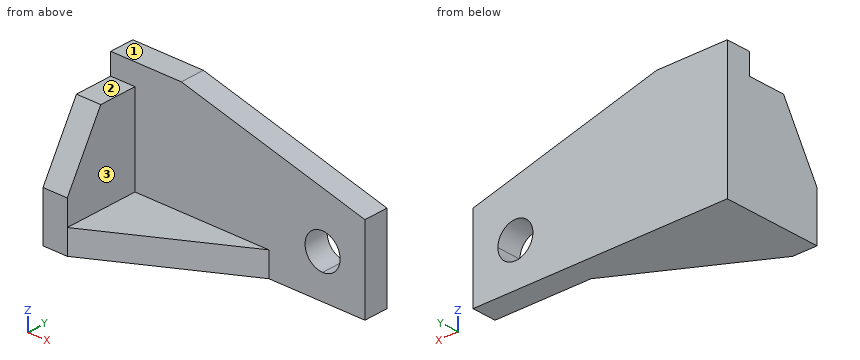
from build123d import *

# Parameters (mm, degrees)
F1_DEPTH  = 10.922
F2_W      = 10.922
F2_H      = 50.8
F3_DEPTH  = 33.528
F4_W      = 60.198
F4_H      = 10.922
F5_DEPTH  = 33.528
F7_DEPTH  = 25.4
F9_DEPTH  = 10.923
F11_DEPTH = 10.923


with BuildPart() as f1:
    # F0 (on Front) → F1 (new body)
    with BuildSketch(Plane.XZ):
        Polygon((-61.109246, 15.510071), (-92.859246, 15.510071), (-92.859246, -44.687929), (21.440754, -44.687929), (21.440754, -6.609135), align=None)
    extrude(amount=F1_DEPTH)

    # F2 (on face) → F3 (join)
    with BuildSketch(Plane.XZ.offset(10.922)):
        with Locations((-87.398246, -19.287929)):
            Rectangle(F2_W, F2_H)
    extrude(amount=F3_DEPTH)

    # F4 (on face) → F5 (join)
    with BuildSketch(Plane.XZ.offset(10.922)):
        with Locations((-51.838246, -39.226929)):
            Rectangle(F4_W, F4_H)
    extrude(amount=F5_DEPTH)

    # F6 (on face) → F7 (cut)
    with BuildSketch(Plane.XY.offset(-33.765929)):
        Polygon((-21.739246, -10.922), (-81.937246, -44.45), (-21.739246, -44.45), align=None)
    extrude(amount=-F7_DEPTH, mode=Mode.SUBTRACT)

    # F8 (on face) → F9 (cut, through all)
    with BuildSketch(Plane.XZ.offset(10.922)):
        with BuildLine():
            ThreePointArc((10.264754, -25.637929), (-3.177005, -20.070171), (2.390754, -33.511929))
            Line((2.390754, -33.511929), (2.390754, -25.637929))
            Line((2.390754, -25.637929), (10.264754, -25.637929))
        make_face()
        with BuildLine():
            Line((2.390754, -25.637929), (2.390754, -33.511929))
            ThreePointArc((2.390754, -33.511929), (7.958513, -31.205688), (10.264754, -25.637929))
            Line((10.264754, -25.637929), (2.390754, -25.637929))
        make_face()
    extrude(amount=-F9_DEPTH, mode=Mode.SUBTRACT)

    # F10 (on face) → F11 (cut, through all)
    with BuildSketch(Plane.YZ.offset(-81.937246)):
        Polygon((-44.45, 6.112071), (-44.45, -22.589929), (-27.878893, 6.112071), align=None)
    extrude(amount=-F11_DEPTH, mode=Mode.SUBTRACT)


solid = f1.part
Read the model definition and answer for the solid it produces. Units are mm, in the model's axes. Face numbers are marked on the shaded views. A direction names the side the tool comes from. Round coordinates to 2 decimals unless told otherwise and drop trailing zeros. Order: outer loops, then holes, each group sorted by start corner. A loop starts at its lowest first (then second) coordinate and runs counter-clockwise, first axis right, second up. Notation, with made-up numbers: (-34, -6) - (3, -6) arc R24 ccw to (3, 6) - close; hole circle Ø5 at (-4.75, 44). An arc over 180 degrees is marked (long way). Use one line per item in the form item = value. Start each with the question number.
(1) The part is cut by section C-C (y = -8). Give the vertices of the cut face in (x, z).
(2) Find the intervals of material crossed by line 1 along Z through (x, y) = (-59.5, -25.5); line 2 along Y through (x, z) = (-15.5, -6); line 3 along X through (y, z) = (-13, -19), in increasing order. Write a range as from..to.
(3) The part is cut by section B-B (z = -32). Give the vertices of the cut face in (x, y).
(4) For the marked faces 1, 2 and 3, determine the directions among +Z, -Z, +X, -X, +Y, -Y from which every point of the face is accessible in a straight line to the end or side of a thin tool.
(5) The part is cut by section A-A (x = 8). Give the vertices of the cut face in (y, z), then the cut area to 3 significant figures.
(6) The part is cut by section D-D (z = -13). Give the vertices of the cut face in (x, y).
(7) Flat-ended cylindrical pins translate along their axes: pin 1 Ø12 at (x, y) = (-51.5, -32) entering from +Z; pin 2 Ø1.5 at (x, z) = (-29.5, -29.5) entering from -Y; pin 3 Ø10 at (y, z) = (-33.5, -22) entering from +X. Find the tip coordinate at first contact, or state that the pin passes through.
Checked values:
q1.outline = (-92.86, -44.69) - (21.44, -44.69) - (21.44, -6.61) - (-61.11, 15.51) - (-92.86, 15.51) - close; hole circle Ø15.75 at (2.39, -25.64)
q2.line_1 = -44.69..-33.77
q2.line_2 = -10.92..0
q2.line_3 = -92.86..-81.94
q3.outline = (-92.86, -44.45) - (-81.94, -44.45) - (-81.94, -10.92) - (-2.25, -10.92) - (-2.25, 0) - (-92.86, 0) - close; (7.03, -10.92) - (21.44, -10.92) - (21.44, 0) - (7.03, 0) - close
q4.face_1 = +Z, +X, -X, +Y, -Y
q4.face_2 = +Z, +X, -X, -Y
q4.face_3 = +Z, +X, -Y
q5.outline = (-10.92, -44.69) - (0, -44.69) - (0, -31.16) - (-10.92, -31.16) - close; (-10.92, -20.11) - (0, -20.11) - (0, -3.01) - (-10.92, -3.01) - close
q5.area = 335 mm^2
q6.outline = (-92.86, -38.91) - (-81.94, -38.91) - (-81.94, -10.92) - (21.44, -10.92) - (21.44, 0) - (-92.86, 0) - close
q7.pin_1 = -33.77
q7.pin_2 = -10.92
q7.pin_3 = -81.94
